Build history of the part. All positions in model axes, mm. A direction names the side the tool comes from. Coordinates: 2 decimals unless noted, no trailing zeros. Order: outer loops, then holes, each group sorted by start corner. A loop starts at its lowest first (then second) coordinate and runs counter-clockwise, first axis right, second up. Notation, with made-up numbers: (-1.75, 32.5) - (35.25, 32.5) arc R9 ccw to (35.25, 45.5) - close; hole circle Ø2 at (38, 18.25). An arc over 180 degrees is marked (long way). Return JSON: item names as keys, results as strings.
from build123d import *

# Parameters (mm, degrees)
SKETCH2_R               = 50.8
BOSS_EXTRUDE1_DEPTH     = 4.7625
BOSS_EXTRUDE2_DEPTH     = 30
CUT_EXTRUDE2_DEPTH      = 128.159272666
CUT_EXTRUDE1_DEPTH      = 111.550805628
CUT_EXTRUDE1_DEPTH_BACK = 111.550805628
SKETCH5_W               = 52
SKETCH5_H               = 33.1537


with BuildPart() as part:
    # Sketch2 → Boss-Extrude1 (new body)
    with BuildSketch(Plane(origin=(0, 37.2625, 0), x_dir=(-1, 0, 0), z_dir=(0, 1, 0))):
        with Locations(Location((0, 0, 0), (0, 0, 270))):
            Circle(SKETCH2_R)
    extrude(amount=BOSS_EXTRUDE1_DEPTH)

    # Sketch4 → Boss-Extrude2 (add, symmetric)
    with BuildSketch(Plane(origin=(0, 0, 0), x_dir=(0, 0, -1), z_dir=(1, 0, 0))):
        Polygon((-25, 42.025), (25, 42.025), (16, 84.025), (-16, 84.025), align=None)
    extrude(amount=BOSS_EXTRUDE2_DEPTH, both=True)

    # Sketch6 → Cut-Extrude2 (cut, through all)
    with BuildSketch(Plane(origin=(30, 0, 0), x_dir=(0, 0, -1), z_dir=(1, 0, 0))):
        with BuildLine():
            Line((5, 78.025), (5, 84.025))
            Line((5, 84.025), (-5, 84.025))
            Line((-5, 84.025), (-5, 78.025))
            ThreePointArc((-5, 78.025), (0, 73.025), (5, 78.025))
        make_face()
    extrude(amount=-CUT_EXTRUDE2_DEPTH, mode=Mode.SUBTRACT)

    # Sketch5 → Cut-Extrude1 (cut, two sides: drawn at the far end of the back side and taken through both)
    with BuildSketch(Plane.XY.offset(-CUT_EXTRUDE1_DEPTH_BACK)):
        with Locations((0, 67.44815)):
            Rectangle(SKETCH5_W, SKETCH5_H)
    extrude(amount=CUT_EXTRUDE1_DEPTH + CUT_EXTRUDE1_DEPTH_BACK, mode=Mode.SUBTRACT)


solid = part.part
1. Cut at B-B on z = 0. Give the cut face in (x, y) (1 decimal), plus the area to 3 significant figures.
Check values:
{"outline": "(-50.8, 37.3) - (50.8, 37.3) - (50.8, 42) - (30, 42) - (30, 73) - (26, 73) - (26, 50.9) - (-26, 50.9) - (-26, 73) - (-30, 73) - (-30, 42) - (-50.8, 42) - close", "area": "1,190 mm²"}
2. Mould opens along X. For faces 1 (the flat face through (28, 84.025, -11)), 2 (the flat face through (-30, 63, 0)), 3 (the flat face through (-26, 64, 0)) say: pulls with the +X half, pulls with the -X half, needs draft (parallel to the pull), parting line crosses it, or undercut.
Check values:
{"face 1": "needs draft", "face 2": "pulls with the -X half", "face 3": "undercut"}
3. Drop flat-ended pins along their axis: pin 1 (2 mm diameter, centred on x = -13.5, z = -21, fed in from +Y); pin 2 (21 mm diameter, centred on y = 72, z = 2.5, fed in from +X); pin 3 (5 mm diameter, centred on y = 42.5, z = -26.5, fed in from +X). Give the stop position or say it passes through.
Check values:
{"pin 1": "y = 50.87", "pin 2": "x = 30", "pin 3": "x = 44.75"}
4. Tool access for faces 4 (the flat face through (33, 42.025, 1)), 5 (the flat face through (0, 50.871, 0)), 6 (the flat face through (28, 81, 5)): list every direction of +Z, -Z, +X, -X, +Y, -Y with a clear straight run to the whole face (end or side of a thin tool).
Check values:
{"face 4": "+Y", "face 5": "+Z, -Z, +Y", "face 6": "+X, -X, +Y"}
5. Cut at A-A on y = 65. Give the cut face in (x, z).
Check values:
{"outline": "(-30, -20.08) - (-26, -20.08) - (-26, 20.08) - (-30, 20.08) - close; (26, -20.08) - (30, -20.08) - (30, 20.08) - (26, 20.08) - close"}
6. Cut at D-D on y = 75. Give the cut face in (x, z), plus the area to 3 significant figures.
Check values:
{"outline": "(-30, -17.93) - (-26, -17.93) - (-26, -3.98) - (-30, -3.98) - close; (-30, 3.98) - (-26, 3.98) - (-26, 17.93) - (-30, 17.93) - close; (26, -17.93) - (30, -17.93) - (30, -3.98) - (26, -3.98) - close; (26, 3.98) - (30, 3.98) - (30, 17.93) - (26, 17.93) - close", "area": "223 mm²"}
7. Probe L1, parallel to X at y = 54.5, z = -12.5; L2, parallel to Y at x = 2.5, z = 5.5; L3, parallel to Y at x = -3.5, z = -37 (1 decimal). List the from-to ranges inside material, lowest first.
Check values:
{"L1": "-30 to -26, 26 to 30", "L2": "37.26 to 50.87", "L3": "37.3 to 42"}
8. Cut at C-C on x = 0. Give the cut face in (y, z) (1 decimal).
Check values:
{"outline": "(37.3, -50.8) - (42, -50.8) - (42, -25) - (50.9, -23.1) - (50.9, 23.1) - (42, 25) - (42, 50.8) - (37.3, 50.8) - close"}
